```python
from build123d import *

# Parameters (mm, degrees)
F1_ANGLE_BACK = 11.25
F1_ANGLE      = 22.5
F2_W          = 174.6602954563
F2_H          = 13.9838710204
F2_W_2        = 174.5945907282
F2_H_2        = 12.7738052979
F3_DEPTH      = 125
F5_DEPTH      = 1.001
F7_DEPTH      = 2.5
F9_DEPTH      = 1
F11_DEPTH     = 2.5
F13_DEPTH     = 2.5


with BuildPart() as f1:
    # F0 (on Front) → F1 (revolve)
    with BuildSketch(Plane.XZ, mode=Mode.PRIVATE) as f1_sk:
        Polygon((4.5, 1.8972494266), (151.4991241063, 1.4046487898), (151.5292833394, 10.4045982575), (4.530159233, 10.8971988943), align=None)
        Polygon((151.4689648733, -7.5953006778), (151.4991241063, 1.4046487898), (4.5, 1.8972494266), (4.4973410418, 1.1037780134), (51.0110905605, -7.2586618498), align=None)
        Polygon((4.469840767, -7.102700041), (51.0110905605, -7.2586618498), (4.4973410418, 1.1037780134), align=None)
    revolve(f1_sk.sketch.rotate(Axis((561.8991869329, 0, -48.7660320647), (-0.176947319, 0, -0.9842203241)), -F1_ANGLE_BACK), axis=Axis((561.8991869329, 0, -48.7660320647), (-0.176947319, 0, -0.9842203241)), revolution_arc=F1_ANGLE)

    # F2 (on Front) → F3 (cut, symmetric)
    with BuildSketch(Plane.XZ):
        with Locations((82.9434095772, 7.9919355102)):
            Rectangle(F2_W, F2_H)
        with Locations((82.9762619412, -6.386902649)):
            Rectangle(F2_W_2, F2_H_2)
    extrude(amount=F3_DEPTH, both=True, mode=Mode.SUBTRACT)

    # F4 (on face) → F5 (cut, through all)
    with BuildSketch(Plane.XY.offset(1)):
        with BuildLine():
            Line((43.4654092359, 97.642850746), (16.9671003359, 102.8305199324))
            ThreePointArc((16.9671003359, 102.8305199324), (7.5, 0), (16.9671003359, -102.8305199324))
            Line((16.9671003359, -102.8305199324), (43.4654092359, -97.642850746))
            ThreePointArc((43.4654092359, -97.642850746), (34.5, 0), (43.4654092359, 97.642850746))
        make_face()
        with BuildLine():
            Line((120.2899679019, 84.1311059323), (52.5732132725, 97.3882584065))
            ThreePointArc((52.5732132725, 97.3882584065), (45.8906345723, 50.1494761623), (43.5059275751, 2.5))
            Line((43.5059275751, 2.5), (112.5068202166, 2.5))
            ThreePointArc((112.5068202166, 2.5), (114.5685951129, 43.4900158167), (120.2899679019, 84.1311059323))
        make_face()
        with BuildLine():
            Line((112.5068202166, -2.5), (43.5059275751, -2.5))
            ThreePointArc((43.5059275751, -2.5), (45.8906345723, -50.1494761623), (52.5732132725, -97.3882584065))
            Line((52.5732132725, -97.3882584065), (120.2899679019, -84.1311059323))
            ThreePointArc((120.2899679019, -84.1311059323), (114.5685951129, -43.4900158167), (112.5068202166, -2.5))
        make_face()
        with BuildLine():
            Line((155.3490104822, 75.7389959439), (128.8499233765, 80.9268174824))
            ThreePointArc((128.8499233765, 80.9268174824), (121.5, 0), (128.8499233765, -80.9268174824))
            Line((128.8499233765, -80.9268174824), (155.3490104822, -75.7389959439))
            ThreePointArc((155.3490104822, -75.7389959439), (148.5, 0), (155.3490104822, 75.7389959439))
        make_face()
    extrude(amount=-F5_DEPTH, mode=Mode.SUBTRACT)

    # F6 (on face) → F7 (join)
    with BuildSketch(Plane.XY.offset(1)):
        Polygon((45.0166627785, 98.8676314601), (45.4585534309, 101.1247829063), (39.5703322667, 102.2775411299), (39.1284416144, 100.0203896837), align=None)
        Polygon((52.5732132725, 97.3882584065), (57.2837902038, 96.4660518276), (57.7064682191, 98.6250662544), (51.818247055, 99.777824478), (51.3955690397, 97.6188100512), align=None)
        Polygon((116.0020689859, 87.2123269381), (115.5793909706, 85.0533125112), (120.2899679019, 84.1311059323), (121.4676121347, 83.9005542876), (121.8902901501, 86.0595687145), align=None)
        Polygon((128.2884090483, 84.908884325), (127.8465183959, 82.6517328787), (133.7347395601, 81.4989746551), (134.1766302124, 83.7561261014), align=None)
        Polygon((120.2899679019, -84.1311059323), (115.5793909706, -85.0533125112), (116.0020689859, -87.2123269381), (121.8902901501, -86.0595687145), (121.4676121347, -83.9005542876), align=None)
        Polygon((133.7347395601, -81.4989746551), (127.8465183959, -82.6517328787), (128.2884090483, -84.908884325), (134.1766302124, -83.7561261014), align=None)
        Polygon((45.4585534309, -101.1247829063), (45.0166627785, -98.8676314601), (39.1284416144, -100.0203896837), (39.5703322667, -102.2775411299), align=None)
        Polygon((57.7064682191, -98.6250662544), (57.2837902038, -96.4660518276), (52.5732132725, -97.3882584065), (51.3955690397, -97.6188100512), (51.818247055, -99.777824478), align=None)
    extrude(amount=F7_DEPTH)

    # F8 (on face) → F9 (join)
    with BuildSketch(Plane.XY.offset(1)):
        Polygon((34.6784961674, 104.9675053569), (17.0138326749, 108.4257800277), (15.9571376366, 103.0282439606), (16.9671003359, 102.8305199324), (33.6218011291, 99.5699692898), align=None)
        Polygon((78.3494698015, 96.4178818652), (63.6289168911, 99.2997774242), (62.8604114087, 95.3742966481), (77.5809643191, 92.4924010891), align=None)
        Polygon((110.7346862043, 90.0777116354), (96.0141332939, 92.9596071944), (95.2456278115, 89.0341264183), (109.9661807219, 86.1522308593), align=None)
        Polygon((157.3497208298, 80.9517187405), (139.6850573373, 84.4099934113), (138.628362299, 79.0124573441), (155.3490104822, 75.7389959439), (156.2930257915, 75.5541826733), align=None)
        Polygon((156.2930257915, -75.5541826733), (155.3490104822, -75.7389959439), (138.628362299, -79.0124573441), (139.6850573373, -84.4099934113), (157.3497208298, -80.9517187405), align=None)
        Polygon((95.2455782208, -89.0341361269), (96.0140837032, -92.959616903), (110.7346366136, -90.077721344), (109.9661311312, -86.1522405679), align=None)
        Polygon((62.860361818, -95.3743063567), (63.6288673004, -99.2997871328), (78.3494202108, -96.4178915738), (77.5809147284, -92.4924107977), align=None)
        Polygon((16.9671003359, -102.8305199324), (14.0205764212, -103.407371511), (15.0510922869, -108.8100327689), (34.6784961674, -104.9675053569), (33.6218011291, -99.5699692898), align=None)
    extrude(amount=F9_DEPTH)

    # F10 (on face) → F11 (join)
    with BuildSketch(Plane(origin=(21.0396507867, -107.4692979953, -3.7825979687), x_dir=(0.9813926052, 0.1918930354, 0.0067540611), z_dir=(0.19201186, -0.9807852804, -0.0345207094))):
        Polygon((-8.8453486731, 3.8468765561), (-6.1087279224, 3.8468765561), (-6.1021027342, 4.826798959), (-5.0953486731, 4.81999507), (-5.0953486731, 5.8261801192), (-5.0953486731, 9.2761801192), (-7.8453486731, 9.2761801192), (-8.8453486731, 4.7761801192), align=None)
        Polygon((-6.1021027342, 4.826798959), (-6.1087279224, 3.8468765561), (-5.0953486731, 3.8468765561), (-5.0953486731, 4.81999507), align=None)
        Polygon((140.8944898216, 3.8333602109), (140.8878160856, 2.8462571659), (143.6378160856, 2.8462571659), (143.6378160856, 3.835607484), (142.6378160856, 8.285607484), (139.8878160856, 8.285607484), (139.8878160856, 4.835607484), (138.0617320538, 4.835607484), (138.474456915, 3.8497153822), (138.8945354939, 3.846876389), align=None)
        Polygon((138.8945354939, 2.8462571659), (140.8878160856, 2.8462571659), (140.8944898216, 3.8333602109), (138.8945354939, 3.846876389), (138.474456915, 3.8497153822), align=None)
    extrude(amount=-F11_DEPTH)

    # F12 (on face) → F13 (join)
    with BuildSketch(Plane(origin=(21.0396507867, 107.4692979953, -3.7825979687), x_dir=(-0.9813926052, 0.1918930354, -0.0067540611), z_dir=(0.19201186, 0.9807852804, -0.0345207094))):
        Polygon((6.1088675431, 3.8262254542), (2.7622254557, 3.8036080325), (4.8167226223, 3.8036080325), (6.1021027342, 3.8036080325), (8.8521027342, 3.8036080325), (8.8521027342, 4.7536080325), (7.8521027342, 9.2536080325), (5.1021027342, 9.2536080325), (5.1021027342, 5.8036080325), (2.7622254557, 5.8036080325), (2.7622254557, 4.8042272555), (4.1021484065, 4.8132827809), (6.1021027342, 4.826798959), align=None)
        Polygon((2.7622254557, 4.8042272555), (2.7622254557, 3.8036080325), (6.1088675431, 3.8262254542), (6.1021027342, 4.826798959), (4.1021484065, 4.8132827809), align=None)
        Polygon((-143.6444898216, 2.832786706), (-140.8877250128, 2.832786706), (-140.8944898216, 3.8333602109), (-138.8945354939, 3.846876389), (-136.8420855995, 3.8607473449), (-136.7184351443, 4.832786706), (-139.8944898216, 4.832786706), (-139.8944898216, 8.282786706), (-142.6444898216, 8.282786706), (-143.6444898216, 3.782786706), align=None)
        Polygon((-140.8944898216, 3.8333602109), (-140.8877250128, 2.832786706), (-136.969481142, 2.8592671517), (-136.8420855995, 3.8607473449), (-138.8945354939, 3.846876389), align=None)
    extrude(amount=-F13_DEPTH)


solid = f1.part
```
Check sheet for the modelled part. Datum: model origin and axes. Units: mm. Coordinates: 2 decimals unless noted, no trailing zeros. Write each loop counter-clockwise with the first axis right and the second up, starting at its lowest first coordinate (ties: lowest second). Pieces come first, ordered by that corner, then holes. Notation, with made-up numbers: (-27, 53) - (22, 53) arc R24 ccw to (22, 69) - close; hole circle Ø4 at (-5.75, 65). An arc over 180 degrees is marked (long way). One line per question, with ' | ' between items.
Item 1: Thickness scan on line 1 (Z direction, x = 43, y = -26.5); line 2 (Y direction, x = 148, z = 0.5); line 3 (Y direction, x = 19, z = 0.35). Record the ranges inside material, lowest first. Write a range as [from, to].
Determined:
line 1: z = [0, 1] | line 2: y = [-82.76, -77.18], [77.18, 82.76] | line 3: y = [-108.01, -102.43], [102.43, 108.01]
Item 2: Sectioned sample at A-A on x = 83. Record the boundary of the cut face in (y, z).
Determined:
outline: (-95.51, 1) - (-95.47, 0) - (-91.43, 0) - (-91.43, 1) - close; (-2.5, 0) - (2.5, 0) - (2.5, 1) - (-2.5, 1) - close; (91.43, 0) - (95.47, 0) - (95.51, 1) - (91.43, 1) - close
Item 3: Sectioned sample at B-B on y = 71.5. Give the number of separate pieces and of enclosed holes in the cut face, plus the area to 3 significant figures.
Determined:
separate pieces: 4 | enclosed holes: 0 | area: 24.3 mm2
Item 4: Gauge pin test, flat ends, axial feed: P1, Ø4, axis at x = 43, y = 100, coming from the +Z side; P2, Ø7, axis at x = 29, y = -102.5, coming from the +Z side; P3, Ø2, axis at x = 40.5, z = 4, coming from the -Y side. Record the tip position at first contact, or that the pin passes through.
Determined:
P1: stops at z = 3.5 | P2: stops at z = 2 | P3: stops at y = -102.27
Item 5: Mould release check, pull along Y, two halves, no side actions. Record for faces 1 (the face through (75, 0, 1)), 2 (the face through (70, 96, 2)): pulls with the +Y half, pulls with the -Y half, needs draft (parallel to the pull), parting line crosses it, or undercut.
Determined:
face 1: undercut | face 2: needs draft
